Input: part model. Units: mm. Frame: model coordinates. Give positions to 0.01 mm unless a question says otherwise; leave off trailing zeros. Loops run counter-clockwise (first coordinate to the right, second up) from the corner with the lowest first, then second, coordinate; pieces in that order, holes last. Notation, with made-up numbers: (55, -0.75) -> (98, -0.75) arc R23 ccw to (98, 34.25) -> close; hole circle Ø8 at (8.25, -28.5). An arc over 180 degrees is marked (long way). Answer as a JSON object with one key per item and string values.
```python
from build123d import *

# Parameters (mm, degrees)
SKETCH1_R           = 80
SKETCH1_R_2         = 60
BOSS_EXTRUDE1_DEPTH = 2.5
SKETCH2_R           = 4
CUT_EXTRUDE1_DEPTH  = 114.247516529
CIRPATTERN1_COUNT   = 20


with BuildPart() as part:
    # Sketch1 → Boss-Extrude1 (new, symmetric)
    with BuildSketch(Plane(origin=(0, 0, 0), x_dir=(0, 0, -1), z_dir=(1, 0, 0))):
        Circle(SKETCH1_R)
        Circle(SKETCH1_R_2, mode=Mode.SUBTRACT)
    extrude(amount=BOSS_EXTRUDE1_DEPTH, both=True)

    # Sketch2 → Cut-Extrude1 (cut, through all)
    with BuildSketch(Plane(origin=(2.5, 0, 0), x_dir=(0, 0, -1), z_dir=(1, 0, 0))):
        with Locations((0, 70)):
            Circle(SKETCH2_R)
        with BuildLine():
            Line((-7.996862967, 55.945192077), (7.996862967, 55.945192077))
            ThreePointArc((7.996862967, 55.945192077), (13.383151066, 60.405313548), (6.750740904, 62.622500611))
            ThreePointArc((6.750740904, 62.622500611), (0, 60), (-6.750740904, 62.622500611))
            ThreePointArc((-6.750740904, 62.622500611), (-13.383151066, 60.405313548), (-7.996862967, 55.945192077))
        make_face()
    cut_extrude1 = extrude(amount=-CUT_EXTRUDE1_DEPTH, mode=Mode.SUBTRACT)

    # CirPattern1: Cut-Extrude1 ×20 about axis
    cirpattern1_axis = Axis((0, 0, 0), (1, 0, 0))
    for i in range(1, CIRPATTERN1_COUNT):
        add(cut_extrude1.rotate(cirpattern1_axis, i * 360 / CIRPATTERN1_COUNT), mode=Mode.SUBTRACT)


solid = part.part
```
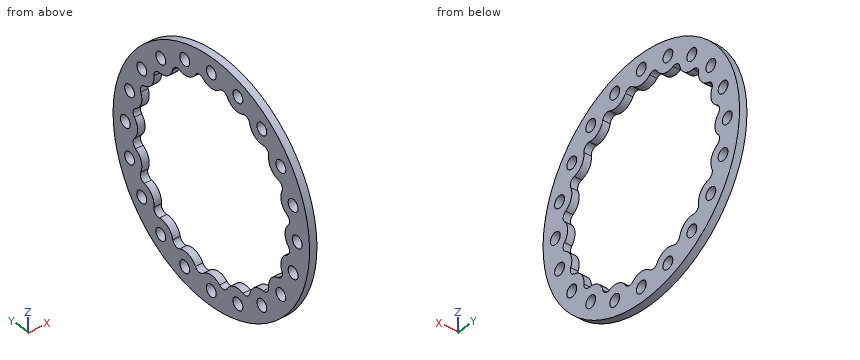
Q1. Section A-A, the plane z = 0. Return the cut outline in (x, y), then the cut area to 3 significant figures.
Evaluation:
{"outline": "(-2.5, -80) -> (2.5, -80) -> (2.5, -74) -> (-2.5, -74) -> close; (-2.5, -66) -> (2.5, -66) -> (2.5, -60) -> (-2.5, -60) -> close; (-2.5, 60) -> (2.5, 60) -> (2.5, 66) -> (-2.5, 66) -> close; (-2.5, 74) -> (2.5, 74) -> (2.5, 80) -> (-2.5, 80) -> close", "area": "120 mm2"}
Q2. Ray query, line 1 along Z through (x, y) = (-1.9, -1); line 2 along Z through (x, y) = (0.9, -22); line 3 along Y through (x, z) = (1.8, 21). Return the intervals inside material, ascending.
Evaluation:
{"line 1": "z = -79.99 to -73.87, -66.13 to -60.05, 60.05 to 66.13, 73.87 to 79.99", "line 2": "z = -76.92 to -70.56, -62.59 to -56.58, 56.58 to 62.59, 70.56 to 76.92", "line 3": "y = -77.19 to -70.52, -62.62 to -56.59, 56.59 to 62.62, 70.52 to 77.19"}
Q3. Section D-D, the plane x = 0.25. Give the number of separate pieces and of enclosed holes in the cut face, then the cut area to 3 significant figures.
Evaluation:
{"separate pieces": "1", "enclosed holes": "21", "area": "7,060 mm2"}
Q4. Pin query (flat end, axial travel): pin 1 (6.5 mm diameter, centred on y = 56.63, z = 41.14, fed in from -X); pin 2 (3 mm diameter, centred on x = -2, y = 60.5, fed in from -Z); pin 3 (3 mm diameter, centred on x = 1, z = 62, fed in from +Y); pin 4 (3 mm diameter, centred on x = -1, y = 46, fed in from -Z). Return the tip coordinate at first contact, or that it passes through.
Evaluation:
{"pin 1": "passes through", "pin 2": "stops at z = -54.03", "pin 3": "stops at y = 52.34", "pin 4": "stops at z = -66.48"}
Q5. Section C-C, the plane y = -33.5. Return the cut outline in (x, z).
Evaluation:
{"outline": "(-2.5, -72.65) -> (2.5, -72.65) -> (2.5, -50.18) -> (-2.5, -50.18) -> close; (-2.5, 50.18) -> (2.5, 50.18) -> (2.5, 72.65) -> (-2.5, 72.65) -> close"}
